For this review, take the finished solid that the model builds, in its own axes (mm). A direction names the side the tool comes from. Coordinates: 2 decimals unless noted, no trailing zeros. Write each loop counter-clockwise with the first axis right and the second up, starting at its lowest first coordinate (ties: lowest second). Pieces come first, ordered by that corner, then holes.
```python
from build123d import *

# Parameters (mm, degrees)
AUFSATZ_LINEAR_AUSTRAGEN1_DEPTH      = 2.5
AUFSATZ_LINEAR_AUSTRAGEN1_DEPTH_BACK = 3
SKIZZE1_W                            = 37.5
SKIZZE1_H                            = 33
SKIZZE2_W                            = 3
SKIZZE2_H                            = 33
SKIZZE2_W_2                          = 8
SKIZZE2_H_2                          = 5.1
AUFSATZ_LINEAR_AUSTRAGEN2_DEPTH      = 12.3
SKIZZE5_R                            = 1.2
SCHNITT_LINEAR_AUSTRAGEN4_DEPTH      = 42.006584837
SKIZZE7_R                            = 1.05
SCHNITT_LINEAR_AUSTRAGEN5_DEPTH      = 10
SKIZZE8_W                            = 5.2
SKIZZE8_H                            = 13
SKIZZE8_W_2                          = 13
SKIZZE8_H_2                          = 5.2
SCHNITT_LINEAR_AUSTRAGEN6_DEPTH      = 2.5
SCHNITT_LINEAR_AUSTRAGEN7_DEPTH      = 30.031922086
SCHNITT_LINEAR_AUSTRAGEN7_DEPTH_BACK = 30.031922086
SKIZZE10_R                           = 1.5
SKIZZE13_R                           = 2.5
SCHNITT_LINEAR_AUSTRAGEN8_DEPTH      = 1.5


with BuildPart() as part:
    # Skizze1 → Aufsatz-Linear austragen1 (new, two sides: drawn at the far end of the back side and taken through both)
    with BuildSketch(Plane(origin=(0, 0, 0), x_dir=(1, 0, 0), z_dir=(0, 1, 0)).offset(-AUFSATZ_LINEAR_AUSTRAGEN1_DEPTH_BACK)):
        Rectangle(SKIZZE1_W, SKIZZE1_H)
    extrude(amount=AUFSATZ_LINEAR_AUSTRAGEN1_DEPTH + AUFSATZ_LINEAR_AUSTRAGEN1_DEPTH_BACK)

    # Skizze2 → Aufsatz-Linear austragen2 (add)
    with BuildSketch(Plane(origin=(0, 2.5, 0), x_dir=(1, 0, 0), z_dir=(0, 1, 0))):
        with Locations((-17.25, 0)):
            Rectangle(SKIZZE2_W, SKIZZE2_H)
        with Locations((0.75, -13.95)):
            Rectangle(SKIZZE2_W_2, SKIZZE2_H_2)
        with Locations((0.75, 13.95)):
            Rectangle(SKIZZE2_W_2, SKIZZE2_H_2)
    extrude(amount=AUFSATZ_LINEAR_AUSTRAGEN2_DEPTH)

    # Skizze5 → Schnitt-Linear austragen4 (cut, through all)
    with BuildSketch(Plane(origin=(-15.75, 0, 0), x_dir=(0, 0, -1), z_dir=(1, 0, 0))):
        with Locations((5.7, 8.65)):
            Circle(SKIZZE5_R)
    extrude(amount=-SCHNITT_LINEAR_AUSTRAGEN4_DEPTH, mode=Mode.SUBTRACT)

    # Skizze7 → Schnitt-Linear austragen5 (cut)
    with BuildSketch(Plane(origin=(4.75, 0, 0), x_dir=(0, 0, -1), z_dir=(1, 0, 0))):
        with Locations((-14.35, 8.65)):
            Circle(SKIZZE7_R)
        with Locations((14.35, 8.65)):
            Circle(SKIZZE7_R)
    extrude(amount=-SCHNITT_LINEAR_AUSTRAGEN5_DEPTH, mode=Mode.SUBTRACT)

    # Skizze8 → Schnitt-Linear austragen6 (cut)
    with BuildSketch(Plane.XZ.offset(3)):
        with Locations((5.277e-06, -12.250005277)):
            Rectangle(SKIZZE8_W, SKIZZE8_H)
        with Locations((12.25, 0)):
            Rectangle(SKIZZE8_W_2, SKIZZE8_H_2)
        with Locations((-12.25, -1.0555e-05)):
            Rectangle(SKIZZE8_W_2, SKIZZE8_H_2)
        with Locations((-5.277e-06, 12.249994723)):
            Rectangle(SKIZZE8_W, SKIZZE8_H)
    extrude(amount=-SCHNITT_LINEAR_AUSTRAGEN6_DEPTH, mode=Mode.SUBTRACT)

    # Skizze10 → Schnitt-Linear austragen7 (cut, two sides: drawn at the far end of the back side and taken through both)
    with BuildSketch(Plane(origin=(0, 0, 0), x_dir=(-1, 0, 0), z_dir=(0, 1, 0)).offset(-SCHNITT_LINEAR_AUSTRAGEN7_DEPTH_BACK)):
        with Locations(Location((-12.25, 0, 0), (0, 0, 90))):
            Circle(SKIZZE10_R)
        with Locations(Location((12.25, 0, 0), (0, 0, 270))):
            Circle(SKIZZE10_R)
    extrude(amount=SCHNITT_LINEAR_AUSTRAGEN7_DEPTH + SCHNITT_LINEAR_AUSTRAGEN7_DEPTH_BACK, mode=Mode.SUBTRACT)

    # Skizze13 → Schnitt-Linear austragen8 (cut)
    with BuildSketch(Plane(origin=(0, 2.5, 0), x_dir=(-1, 0, 0), z_dir=(0, 1, 0))):
        with Locations(Location((12.25, 0, 0), (0, 0, 90))):
            Circle(SKIZZE13_R)
        with Locations(Location((-12.25, 0, 0), (0, 0, 270))):
            Circle(SKIZZE13_R)
    extrude(amount=-SCHNITT_LINEAR_AUSTRAGEN8_DEPTH, mode=Mode.SUBTRACT)


solid = part.part
```
1) Consider section B-B (x = -12.25). Give the boundary of the cut face in (y, z).
2) Consider section D-D (z = 0). Give the boundary of the cut face in (x, y).
3) For L1, parallel to X at y = 0.25, z = 0; L2, parallel to X at y = 1.9, z = 0; L3, parallel to Z at x = 12.25, y = 1.8, list the stretches that pass through material, from the lowest coordinate up.
4) Consider section C-C (z = -14.35). Give the boundary of the cut face in (x, y), then the cut area to 3 significant figures.
5) Consider section A-A (y = 8.65). Give the boundary of the cut face in (x, z), then the cut area to 3 significant figures.
6) Tool access review of faces 1 (the face through (4.75, 9, 13)), 2 (the face through (0.8, 8.7, 15.4)), 3 (the face through (0, -0.5, 11)): name each direction out of +Z, -Z, +X, -X, +Y, -Y from which nothing blocks a thin tool from reaching the whole face with its end or side.
7) The part is to be moulded in two halves that separate along Y. For faces 4 (the face through (-17.229, 9.461, -4.816)), 5 (the face through (1, 2.5, 0)), 6 (the face through (12, -2, -2.6)), say which applies: pulls with the +Y half, pulls with the -Y half, needs draft (parallel to the pull), parting line crosses it, or undercut.
8) Clearance check with flat-ended pins moving along their axes: P1, Ø10, axis at x = 1, z = 3, coming from the +Y side; P2, Ø5, axis at x = -15, z = -2.5, coming from the +Y side; P3, Ø3.5, axis at x = -12.25, z = 0, coming from the +Y side; P4, Ø2.5, axis at x = 0.5, z = 12.5, coming from the -Y side. State where each tip first meets the part, or that it passes through.
Results:
1. outline: (-3, -16.5) - (2.5, -16.5) - (2.5, -2.5) - (1, -2.5) - (1, -1.5) - (-0.5, -1.5) - (-0.5, -2.6) - (-3, -2.6) - close; (-3, 2.6) - (-0.5, 2.6) - (-0.5, 1.5) - (1, 1.5) - (1, 2.5) - (2.5, 2.5) - (2.5, 16.5) - (-3, 16.5) - close
2. outline: (-18.75, -0.5) - (-13.75, -0.5) - (-13.75, 1) - (-14.75, 1) - (-14.75, 2.5) - (-15.75, 2.5) - (-15.75, 14.8) - (-18.75, 14.8) - close; (-10.75, -0.5) - (-5.75, -0.5) - (-5.75, -3) - (5.75, -3) - (5.75, -0.5) - (10.75, -0.5) - (10.75, 1) - (9.75, 1) - (9.75, 2.5) - (-9.75, 2.5) - (-9.75, 1) - (-10.75, 1) - close; (13.75, -0.5) - (18.75, -0.5) - (18.75, 2.5) - (14.75, 2.5) - (14.75, 1) - (13.75, 1) - close
3. L1: x = -18.75 to -13.75, -10.75 to 10.75, 13.75 to 18.75
3. L2: x = -18.75 to -14.75, -9.75 to 9.75, 14.75 to 18.75
3. L3: z = -16.5 to -2.5, 2.5 to 16.5
4. outline: (-18.75, -3) - (-2.6, -3) - (-2.6, -0.5) - (2.6, -0.5) - (2.6, -3) - (18.75, -3) - (18.75, 2.5) - (4.75, 2.5) - (4.75, 7.6) - (-3.25, 7.6) - (-3.25, 2.5) - (-15.75, 2.5) - (-15.75, 14.8) - (-18.75, 14.8) - close; (-3.25, 9.7) - (4.75, 9.7) - (4.75, 14.8) - (-3.25, 14.8) - close
4. area: 312 mm2
5. outline: (-18.75, -16.5) - (-15.75, -16.5) - (-15.75, -6.9) - (-18.75, -6.9) - close; (-18.75, -4.5) - (-15.75, -4.5) - (-15.75, 16.5) - (-18.75, 16.5) - close; (-3.25, -16.5) - (4.75, -16.5) - (4.75, -15.4) - (-3.25, -15.4) - close; (-3.25, -13.3) - (4.75, -13.3) - (4.75, -11.4) - (-3.25, -11.4) - close; (-3.25, 11.4) - (4.75, 11.4) - (4.75, 13.3) - (-3.25, 13.3) - close; (-3.25, 15.4) - (4.75, 15.4) - (4.75, 16.5) - (-3.25, 16.5) - close
5. area: 140 mm2
6. face 1: +Z, -Z, +X, +Y
6. face 2: +X
6. face 3: +Z, -Y
7. face 4: undercut
7. face 5: pulls with the +Y half
7. face 6: needs draft
8. P1: stops at y = 2.5
8. P2: stops at y = 14.8
8. P3: stops at y = 1
8. P4: stops at y = -0.5
